Input: part model. Units: mm. Frame: model coordinates. Face numbers are marked on the shaded views. Round coordinates to 2 decimals unless told otherwise and drop trailing zeros. Order: outer loops, then holes, each group sorted by start corner. A loop starts at its lowest first (then second) coordinate and runs counter-clockwise, first axis right, second up. Notation, with made-up numbers: (76.5, 7) - (94.5, 7) arc R16 ccw to (94.5, 18) - close; hole circle Ø11 at (12.25, 62). An arc over 180 degrees is marked (long way). One line per item, written item: value. Start each with the question number.
from build123d import *

# Parameters (mm, degrees)
F0_R     = 9.75
F0_R_2   = 8.1
F1_DEPTH = 43
F2_SIZE  = 0.3


with BuildPart() as f1:
    # F0 (on Top) → F1 (new body)
    with BuildSketch(Plane.XY):
        Circle(F0_R)
        Circle(F0_R_2, mode=Mode.SUBTRACT)
    extrude(amount=F1_DEPTH)

    # F2
    f2_edges = [f1.edges().sort_by_distance(p)[0] for p in [
        (9.75, 0, 21.5),
        (-9.75, 0, 0),
        (-9.75, 0, 43),
        (8.1, 0, 21.5),
        (-8.1, 0, 0),
        (-8.1, 0, 43),
    ]]
    chamfer(f2_edges, length=F2_SIZE)


solid = f1.part
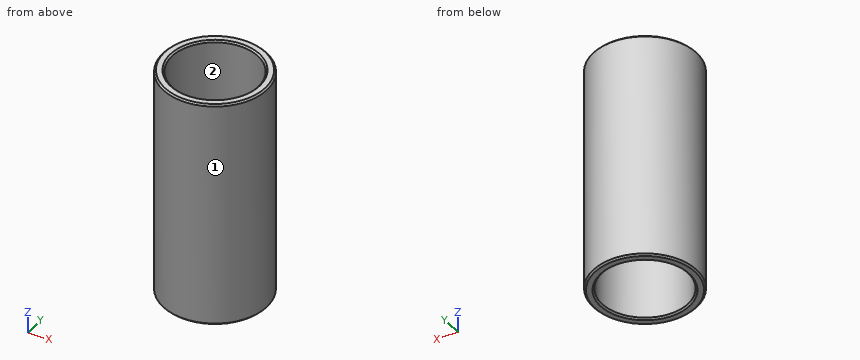
1. Section C-C (z = 12). Return the cut outline in (x, y).
2. Line query: line 1 (Y direction, x = 0, z = 29); line 2 (X direction, y = 7, z = 37); line 3 (Y direction, x = -4, z = 33). Output: solid intervals per line, ascending. Write a range as from..to.
3. Section A-A (y = 0). Return the cut outline in (x, z), then the cut area to 3 significant figures.
4. Pin query (flat end, axial travel): pin 1 (4 mm diameter, centred on x = -5.5, z = 36, fed in from -Y); pin 2 (2 mm diameter, centred on x = 6, z = 26, fed in from +Y); pin 3 (10 mm diameter, centred on y = 6.5, z = 36, fed in from +X). Return the tip coordinate at first contact, or that it passes through.
5. Pull-direction query (X, two-part tool) for the marked faces 1 and 2; classes: released by +X, released by -X, zero draft, split by the parting line, or undercut.
Solved:
1. outline: circle Ø19.5 at (0, 0); hole circle Ø16.2 at (0, 0)
2. line 1: y = -9.75..-8.1, 8.1..9.75
2. line 2: x = -6.79..-4.08, 4.08..6.79
2. line 3: y = -8.89..-7.04, 7.04..8.89
3. outline: (-9.75, 0.3) - (-9.45, 0) - (-8.4, 0) - (-8.1, 0.3) - (-8.1, 42.7) - (-8.4, 43) - (-9.45, 43) - (-9.75, 42.7) - close; (8.1, 0.3) - (8.4, 0) - (9.45, 0) - (9.75, 0.3) - (9.75, 42.7) - (9.45, 43) - (8.4, 43) - (8.1, 42.7) - close
3. area: 142 mm²
4. pin 1: stops at y = -9.1
4. pin 2: stops at y = 8.37
4. pin 3: stops at x = 9.63
5. face 1: split by the parting line
5. face 2: undercut
